from build123d import *

# Parameters (mm, degrees)
F0_W           = 38.1
F0_H           = 101.6
F1_DEPTH       = 3.175
F3_D           = 4.9784
F3_CSINK_D     = 9.1186
F3_CSINK_ANGLE = 82


# Not quite as in the source:
# - a feature names something its author has since deleted; it is built from what else it names


with BuildPart() as f1:
    # F0 (on Right) → F1 (new body)
    with BuildSketch(Plane.YZ):
        Rectangle(F0_W, F0_H)
    extrude(amount=F1_DEPTH)

    # F3 (through all)
    with Locations(Plane.YZ.offset(3.175)):
        with Locations((-9.525, 41.275), (9.525, -41.275)):
            CounterSinkHole(F3_D / 2, F3_CSINK_D / 2, counter_sink_angle=F3_CSINK_ANGLE)


solid = f1.part
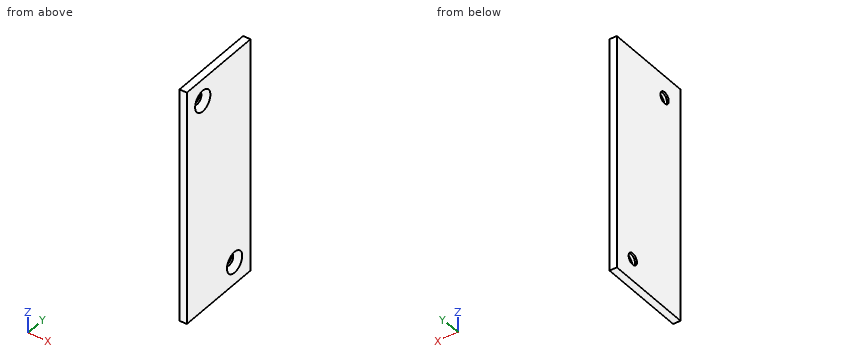
For this review, take the finished solid that the model builds, in its own axes (mm). Round coordinates to 2 decimals unless told otherwise and drop trailing zeros. Loops run counter-clockwise (first coordinate to the right, second up) from the corner with the lowest first, then second, coordinate; pieces in that order, holes last. Notation, with made-up numbers: (0.25, -32.75) - (4.25, -32.75) arc R23 cw to (4.25, -17.75) - close; hole circle Ø3 at (61.25, 81). An arc over 180 degrees is marked (long way). Answer as CSV lines item,"result".
(1) Wall thickness on line 1 (Z direction, x = 1.4, y = 12); line 2 (Y direction, x = 1.1, z = 41); line 3 (Z direction, x = 2.75, y = 7): over which ranges is each line inside the solid? List them lowest first.
Checked values:
line 1,"z = -50.8 to -43, -39.55 to 50.8"
line 2,"y = -19.05 to -12.27, -6.78 to 19.05"
line 3,"z = -50.8 to -44.62, -37.93 to 50.8"
(2) Consider section A-A on x = 1.8. Give the boundary of the cut face in (y, z) (3 decimals).
Checked values:
outline,"(-19.05, -50.8) - (19.05, -50.8) - (19.05, 50.8) - (-19.05, 50.8) - close; hole circle Ø6.728 at (-9.525, 41.275); hole circle Ø6.728 at (9.525, -41.275)"
(3) Insertion check: P1, Ø4, axis at y = 9.525, z = -41.275, coming from the -X side; P2, Ø6.5, axis at y = -9.525, z = 41.275, coming from the +X side. Each pin has a flat end and moves straight along its axis. Give the tip position at first contact, or say it passes through.
Checked values:
P1,"passes through"
P2,"stops at x = 1.67"
